Geometry: final body of the model. Coordinates: model frame, mm. A direction names the side the tool comes from. Give positions to 0.01 mm unless a question says otherwise; leave off trailing zeros. Order: outer loops, then holes, each group sorted by start corner. A loop starts at its lowest first (then second) coordinate and runs counter-clockwise, first axis right, second up. Notation, with made-up numbers: (10.5, 53) -> (54.5, 53) arc R17 cw to (54.5, 84) -> close; hole circle Ø1 at (-25.5, 51). An arc over 180 degrees is marked (long way). One line per question, with ' | ' between items. Start each with the question number.
(1) Mould query, pull axis X, two halves, no side actions, for faces 1 (the face through (-1, 20, -1)), 2 (the face through (-75, 10, 1)), 3 (the face through (-43.494, 10.14, 0.044)). Classes: +X half, -X half, draft (parallel to the pull), parting line (faces both ways), or undercut.
(2) Section A-A (x = -38). Return loops of the section in (y, z), then the cut area to 3 significant figures.
(3) Section B-B (y = 18.25). State how many separate pieces and enclosed holes the cut face has, then the cut area to 3 significant figures.
(4) Ray query, L1, parallel to Z at x = 38, y = 17.3; L2, parallel to Z at x = 29.5, y = 17.75; L3, parallel to Y at x = -35, z = 0. Return the intervals inside material, ascending.
(5) First-contact query: pin 1 Ø10 at (x, z) = (-32.5, -32) entering from -Y. Flat tip, straight axial feed; report the tip coordinate or a pass-through.
(6) Set-up query: faces 4 (the face through (38, 15, 0)), 5 (the face through (-1, 10, 45)), 6 (the face through (38, 10, 12)). Return all of +Z, -Z, +X, -X, +Y, -Y with unobstructed straight access to the full face (end or side cutting, diameter ignored); none if empty.
```python
from build123d import *

# Parameters (mm, degrees)
SKETCH2_W           = 150
SKETCH2_H           = 90
BOSS_EXTRUDE1_DEPTH = 20
SKETCH3_R           = 4
CUT_EXTRUDE1_DEPTH  = 5
CUT_EXTRUDE2_DEPTH  = 21


with BuildPart() as part:
    # Sketch2 → Boss-Extrude1 (new body)
    with BuildSketch(Plane(origin=(0, 0, 0), x_dir=(1, 0, 0), z_dir=(0, 1, 0))):
        Rectangle(SKETCH2_W, SKETCH2_H)
    extrude(amount=BOSS_EXTRUDE1_DEPTH)

    # Sketch3 → Cut-Extrude1 (cut)
    with BuildSketch(Plane(origin=(0, 20, 0), x_dir=(1, 0, 0), z_dir=(0, 1, 0))):
        with Locations((-38, 0)):
            Circle(SKETCH3_R)
        with Locations((38, 0)):
            Circle(SKETCH3_R)
    extrude(amount=-CUT_EXTRUDE1_DEPTH, mode=Mode.SUBTRACT)

    # Sketch4 → Cut-Extrude2 (cut, through all)
    with BuildSketch(Plane(origin=(0, 20, 0), x_dir=(1, 0, 0), z_dir=(0, 1, 0))):
        with BuildLine():
            Line((-45.5, 2.006446443), (-48, 2.006446443))
            ThreePointArc((-48, 2.006446443), (-50.006446443, 0), (-48, -2.006446443))
            Line((-48, -2.006446443), (-45.5, -2.006446443))
            ThreePointArc((-45.5, -2.006446443), (-43.493553557, 0), (-45.5, 2.006446443))
        make_face()
        with BuildLine():
            Line((-36, 7.5), (-36, 10))
            ThreePointArc((-36, 10), (-38, 12), (-40, 10))
            Line((-40, 10), (-40, 7.5))
            ThreePointArc((-40, 7.5), (-38, 5.5), (-36, 7.5))
        make_face()
        with BuildLine():
            Line((-28, 2), (-30.5, 2))
            ThreePointArc((-30.5, 2), (-32.5, 0), (-30.5, -2))
            Line((-30.5, -2), (-28, -2))
            ThreePointArc((-28, -2), (-26, 0), (-28, 2))
        make_face()
        with BuildLine():
            Line((-40, -7.5), (-40, -10))
            ThreePointArc((-40, -10), (-38, -12), (-36, -10))
            Line((-36, -10), (-36, -7.5))
            ThreePointArc((-36, -7.5), (-38, -5.5), (-40, -7.5))
        make_face()
        with BuildLine():
            ThreePointArc((48, -2.006446443), (50.006446443, 0), (48, 2.006446443))
            Line((48, 2.006446443), (45.5, 2.006446443))
            ThreePointArc((45.5, 2.006446443), (43.493553557, 0), (45.5, -2.006446443))
            Line((45.5, -2.006446443), (48, -2.006446443))
        make_face()
        with BuildLine():
            ThreePointArc((40, 10), (38, 12), (36, 10))
            Line((36, 10), (36, 7.5))
            ThreePointArc((36, 7.5), (38, 5.5), (40, 7.5))
            Line((40, 7.5), (40, 10))
        make_face()
        with BuildLine():
            ThreePointArc((30.5, -2), (32.5, 0), (30.5, 2))
            Line((30.5, 2), (28, 2))
            ThreePointArc((28, 2), (26, 0), (28, -2))
            Line((28, -2), (30.5, -2))
        make_face()
        with BuildLine():
            ThreePointArc((36, -10), (38, -12), (40, -10))
            Line((40, -10), (40, -7.5))
            ThreePointArc((40, -7.5), (38, -5.5), (36, -7.5))
            Line((36, -7.5), (36, -10))
        make_face()
    extrude(amount=-CUT_EXTRUDE2_DEPTH, mode=Mode.SUBTRACT)


solid = part.part
```
Response:
1) face 1: draft | face 2: -X half | face 3: undercut
2) outline: (0, -45) -> (20, -45) -> (20, -12) -> (0, -12) -> close; (0, -5.5) -> (20, -5.5) -> (20, -4) -> (15, -4) -> (15, 4) -> (20, 4) -> (20, 5.5) -> (0, 5.5) -> close; (0, 12) -> (20, 12) -> (20, 45) -> (0, 45) -> close | area: 1,500 mm^2
3) separate pieces: 1 | enclosed holes: 10 | area: 13,200 mm^2
4) L1: z = -45 to -12, -5.5 to -4, 4 to 5.5, 12 to 45 | L2: z = -45 to -2, 2 to 45 | L3: y = 0 to 15
5) pin 1: stops at y = 0
6) face 4: +Y | face 5: +Z, +X, -X, +Y, -Y | face 6: +Y, -Y
